Study the drawing (mm; zero at the part's minimum x, y, z) and answer. A direction names the side the tool comes from. Round coordinates to 2 decimals unless told otherwise and drop trailing zeros. Order: outer loops, then holes, each group sorted by start corner. A loop starts at its lowest first (then second) coordinate and runs counter-clockwise, first axis right, second up. Notation, with made-up numbers: (-18.75, 28.25) - (27.25, 28.25) arc R20 ccw to (27.25, 51.25) - close; hole circle Ø11 at (45.25, 27). An arc over 180 degrees is marked (long way). Put each result on its own line as item: value. Start each with the question number.
Q1. Section D-D on x = 30.5 is taken. Give the vertices of the cut face in (y, z) (1 decimal).
Q2. This flat-tipped pin is pushed along its axis until it touches: pin 1 Ø1.5 at (x, z) = (15, 4) entering from -Y. Where does it stop, or does it pass through?
Q3. Which of the six approach directions +Z, -Z, +X, -X, +Y, -Y give full straight-line access (tool end or side, diameter ignored) to the marked faces 4, 5 and 6?
Q4. Section B-B on x = 23 is taken. Give the vertices of the cut face in (y, z) (1 decimal), then the cut area to 3 significant figures.
Q5. Find the intervals of material crossed by line 1 along Y through (x, z) = (16, 3.05); line 2 along X through (y, z) = (6.5, 3.7); line 3 along X through (y, z) = (11.25, 2.5), in increasing order. Write a range as from..to.
Q6. Section C-C on y = 10 is taken. Give the vertices of the cut face in (x, z) (1 decimal).
Q7. For a pull along Y with two mould halves and no side action, classify the marked faces 1, 2 and 3 as pulls with the +Y half, pulls with the -Y half, needs draft (parallel to the pull), parting line crosses it, or undercut.
Q8. Section A-A on z = 1.4 is taken. Give the vertices of the cut face in (x, y) (1 decimal), then the cut area to 3 significant figures.
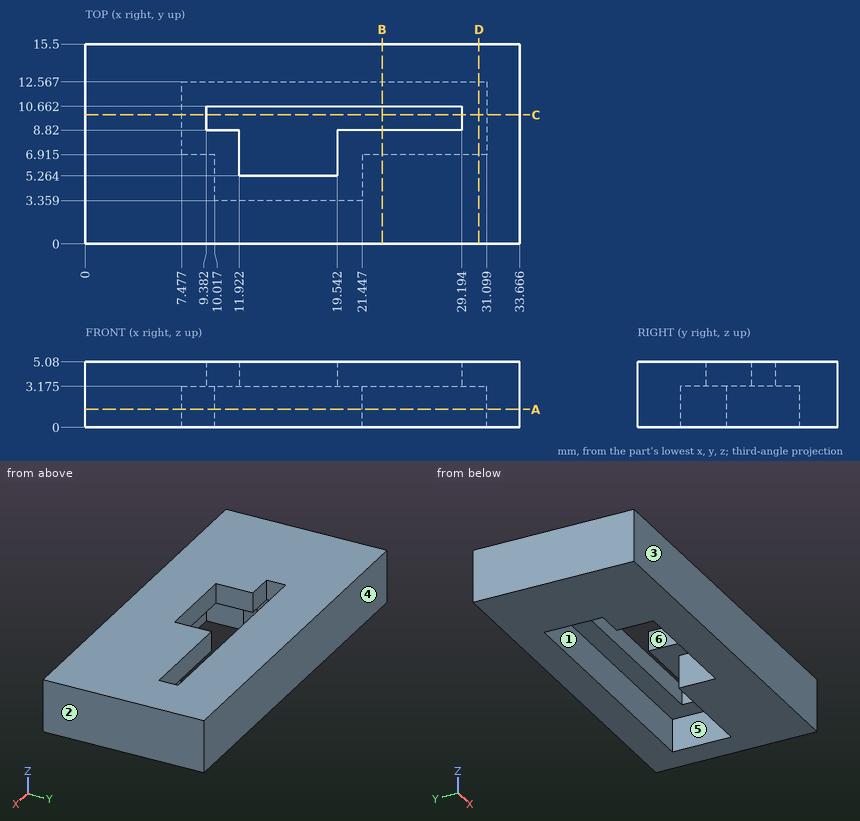
Findings:
1. outline: (0, 0) - (6.9, 0) - (6.9, 3.2) - (12.6, 3.2) - (12.6, 0) - (15.5, 0) - (15.5, 5.1) - (0, 5.1) - close
2. pin 1: y = 0
3. face 4: +Z, -Z, +X, -X, +Y
3. face 5: -Z
3. face 6: +Z, -Z
4. outline: (0, 0) - (6.9, 0) - (6.9, 3.2) - (8.8, 3.2) - (8.8, 5.1) - (0, 5.1) - close; (10.7, 3.2) - (12.6, 3.2) - (12.6, 0) - (15.5, 0) - (15.5, 5.1) - (10.7, 5.1) - close
4. area: 57.3 mm2
5. line 1: 0..3.36, 12.57..15.5
5. line 2: 0..11.92, 19.54..33.67
5. line 3: 0..7.48, 31.1..33.67
6. outline: (0, 0) - (7.5, 0) - (7.5, 3.2) - (9.4, 3.2) - (9.4, 5.1) - (0, 5.1) - close; (29.2, 3.2) - (31.1, 3.2) - (31.1, 0) - (33.7, 0) - (33.7, 5.1) - (29.2, 5.1) - close
7. face 1: undercut
7. face 2: needs draft
7. face 3: pulls with the -Y half
8. outline: (0, 0) - (33.7, 0) - (33.7, 15.5) - (0, 15.5) - close; hole (7.5, 6.9) - (10, 6.9) - (10, 3.4) - (21.4, 3.4) - (21.4, 6.9) - (31.1, 6.9) - (31.1, 12.6) - (7.5, 12.6) - close
8. area: 348 mm2
